Can you work these out from the model? Positions are in its coordinate system, mm. Face numbers are marked on the shaded views. A direction names the side the tool comes from. Coordinates: 2 decimals unless noted, no trailing zeros. Order: outer loops, then holes, each group sorted by start corner. A loop starts at its lowest first (then second) coordinate and runs counter-clockwise, first axis right, second up. Notation, with made-up numbers: M 58.25,-12.75 L 68.25,-12.75 A35 cw 68.25,20.25 Z; hole C 35.5,61 d9. An arc over 180 degrees is marked long. Answer as CSV lines item,"result". Start each with the question number.
1. I need wall thicknesses on line 1 along Y through (x, z) = (22.5, -10); line 2 along X through (y, z) = (34, -7.5); line 3 along Y through (x, z) = (14.75, -5). Which ranges of each line are inside material? Lowest first, please. Write a range as from..to.
2. If we mould it in two halves opening along Y, with no side actions, what happens to the marked faces 3, 4 and 5? For each: released by +Y, released by -Y, zero draft, split by the parting line, or undercut.
3. If we section it at B-B (z = -9): List the corners of the cut face in (x, y) for me.
4. On a 3-axis mill with a long thin cutter (end or side, diameter ignored), from which of +Z, -Z, +X, -X, +Y, -Y can I reach the whole of each face in a straight line? I mean the marked faces 1 and 2. Say none if no direction works.
5. If we section it at C-C (x = 8): List the corners of the cut face in (y, z) for me, plus the area to 3 significant figures.
6. If we section it at D-D (y = 5): List the corners of the cut face in (x, z) for me, plus the area to 3 significant figures.
7. Will this pin go through, and if not, where does the flat tip stop? pin 1 (1 mm diameter, centred on x = 21.5, y = 38, fed in from +Z).
8. If we section it at A-A (y = 34): List the corners of the cut face in (x, z) for me.
```python
from build123d import *

# Parameters (mm, degrees)
SKETCH_3_W          = 26.8
SKETCH_3_H          = 39.8
EXTRUDE_3_DEPTH     = 11
SKETCH_3_3_W        = 24.8
SKETCH_3_3_H        = 34
SKETCH_3_3_W_2      = 9
SKETCH_3_3_H_2      = 3.4
CUT_EXTRUDE_1_DEPTH = 10.2
SKETCH_3_4_W        = 3
SKETCH_3_4_H        = 5
CUT_EXTRUDE_2_DEPTH = 3
SKETCH_3_5_W        = 2.5
SKETCH_3_5_H        = 0.8
CUT_EXTRUDE_3_DEPTH = 3
SKETCH_3_6_W        = 1.2
SKETCH_3_6_H        = 0.8
CUT_EXTRUDE_4_DEPTH = 3
SKETCH_3_7_W        = 1.2
SKETCH_3_7_H        = 0.8
CUT_EXTRUDE_5_DEPTH = 1.5
EXTRUDE_4_DEPTH     = 6
FILLET_1_R          = 1.4
FILLET_2_R          = 1.2
FILLET_3_R          = 0.5


with BuildPart() as part:
    # Sketch 3 → Extrude 3 (new body)
    with BuildSketch(Plane.XY):
        with Locations((13.4, 19.9)):
            Rectangle(SKETCH_3_W, SKETCH_3_H)
    extrude(amount=-EXTRUDE_3_DEPTH)

    # Sketch 3_3 → Cut-Extrude 1 (cut)
    with BuildSketch(Plane.XY):
        with Locations((13.4, 17.8)):
            Rectangle(SKETCH_3_3_W, SKETCH_3_3_H)
        with Locations((21.3, 37.3)):
            Rectangle(SKETCH_3_3_W_2, SKETCH_3_3_H_2)
        Polygon((11.8, 38.1), (11.8, 35.6), (13, 35.6), (16.8, 35.6), (16.8, 38.1), align=None)
    extrude(amount=-CUT_EXTRUDE_1_DEPTH, mode=Mode.SUBTRACT)

    # Sketch 3_4 → Cut-Extrude 2 (cut)
    with BuildSketch(Plane.XY):
        with Locations((4.5, 37.3)):
            Rectangle(SKETCH_3_4_W, SKETCH_3_4_H)
    extrude(amount=-CUT_EXTRUDE_2_DEPTH, mode=Mode.SUBTRACT)

    # Sketch 3_5 → Cut-Extrude 3 (cut)
    with BuildSketch(Plane.XY):
        with Locations((4.25, 0.4)):
            Rectangle(SKETCH_3_5_W, SKETCH_3_5_H)
        with Locations((9.75, 0.4)):
            Rectangle(SKETCH_3_5_W, SKETCH_3_5_H)
    extrude(amount=-CUT_EXTRUDE_3_DEPTH, mode=Mode.SUBTRACT)

    # Sketch 3_6 → Cut-Extrude 4 (cut)
    with BuildSketch(Plane.XY):
        with Locations((23.2, 0.4)):
            Rectangle(SKETCH_3_6_W, SKETCH_3_6_H)
    extrude(amount=-CUT_EXTRUDE_4_DEPTH, mode=Mode.SUBTRACT)

    # Sketch 3_7 → Cut-Extrude 5 (cut)
    with BuildSketch(Plane.XY):
        with Locations((12.4, 35.2)):
            Rectangle(SKETCH_3_7_W, SKETCH_3_7_H)
    extrude(amount=-CUT_EXTRUDE_5_DEPTH, mode=Mode.SUBTRACT)

    # Sketch 4 → Extrude 4 (add)
    with BuildSketch(Plane.XY.offset(-10.2)):
        with BuildLine():
            Line((10.4, 34.8), (16.4, 34.8))
            Line((16.4, 34.8), (16.4, 33.415875518))
            ThreePointArc((16.4, 33.415875518), (16.341421356, 33.274454162), (16.2, 33.215875518))
            Line((16.2, 33.215875518), (10.6, 33.215875518))
            ThreePointArc((10.6, 33.215875518), (10.458578644, 33.274454162), (10.4, 33.415875518))
            Line((10.4, 33.415875518), (10.4, 34.8))
        make_face()
        with BuildLine():
            Line((1, 0.8), (2, 0.8))
            Line((2, 0.8), (2, 1.6))
            ThreePointArc((2, 1.6), (1.941421356, 1.741421356), (1.8, 1.8))
            Line((1.8, 1.8), (1, 1.8))
            Line((1, 1.8), (1, 0.8))
        make_face()
        with BuildLine():
            Line((25.8, 0.8), (24.8, 0.8))
            Line((24.8, 0.8), (24.8, 1.6))
            ThreePointArc((24.8, 1.6), (24.858578644, 1.741421356), (25, 1.8))
            Line((25, 1.8), (25.8, 1.8))
            Line((25.8, 1.8), (25.8, 0.8))
        make_face()
    extrude(amount=EXTRUDE_4_DEPTH)

    # Fillet 1
    fillet_1_edges = [part.edges().sort_by_distance(p)[0] for p in [
        (3, 37.3, -3),
        (6, 37.3, -3),
    ]]
    fillet(fillet_1_edges, radius=FILLET_1_R)

    # Fillet 2
    fillet_2_edges = [part.edges().sort_by_distance(p)[0] for p in [
        (3, 0.4, -3),
        (5.5, 0.4, -3),
        (8.5, 0.4, -3),
        (11, 0.4, -3),
    ]]
    fillet(fillet_2_edges, radius=FILLET_2_R)

    # Fillet 3
    fillet_3_edges = [part.edges().sort_by_distance(p)[0] for p in [
        (23.8, 0.4, -3),
        (11.8, 35.2, -1.5),
        (13, 35.2, -1.5),
        (22.6, 0.4, -3),
    ]]
    fillet(fillet_3_edges, radius=FILLET_3_R)


solid = part.part
```
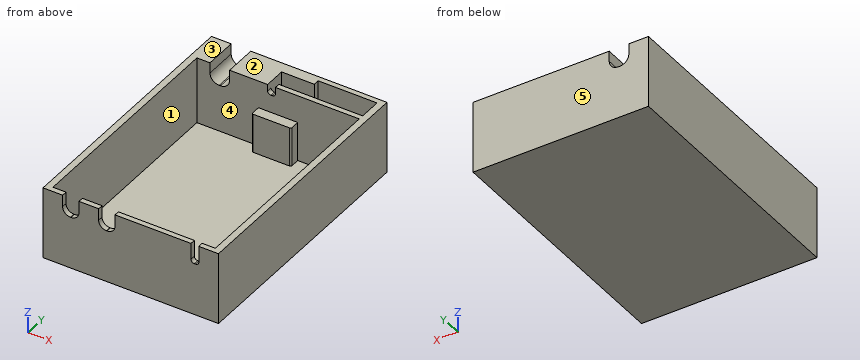
Solved:
1,line 1,"0..0.8, 34.8..35.6, 39..39.8"
1,line 2,"0..1, 10.4..16.4, 25.8..26.8"
1,line 3,"0..0.8, 33.22..35.6, 38.1..39.8"
2,face 3,"zero draft"
2,face 4,"undercut"
2,face 5,"released by +Y"
3,outline,"M 0,0 L 26.8,0 L 26.8,39.8 L 0,39.8 Z; hole M 1,1.8 L 1.8,1.8 A0.2 cw 2,1.6 L 2,0.8 L 24.8,0.8 L 24.8,1.6 A0.2 cw 25,1.8 L 25.8,1.8 L 25.8,34.8 L 16.4,34.8 L 16.4,33.42 A0.2 cw 16.2,33.22 L 10.6,33.22 A0.2 cw 10.4,33.42 L 10.4,34.8 L 1,34.8 Z; hole M 11.8,35.6 L 25.8,35.6 L 25.8,39 L 16.8,39 L 16.8,38.1 L 11.8,38.1 Z"
4,face 1,"+Z"
4,face 2,"+Z, +X, -X, +Y, -Y"
5,outline,"M 0,-11 L 39.8,-11 L 39.8,0 L 34.8,0 L 34.8,-10.2 L 0.8,-10.2 L 0.8,0 L 0,0 Z"
5,area,"91.0 mm²"
6,outline,"M 0,-11 L 26.8,-11 L 26.8,0 L 25.8,0 L 25.8,-10.2 L 1,-10.2 L 1,0 L 0,0 Z"
6,area,"41.8 mm²"
7,pin 1,"z = -10.2"
8,outline,"M 0,-11 L 26.8,-11 L 26.8,0 L 25.8,0 L 25.8,-10.2 L 16.4,-10.2 L 16.4,-4.2 L 10.4,-4.2 L 10.4,-10.2 L 1,-10.2 L 1,0 L 0,0 Z"
